Can you work these out from the model? Positions are in its coordinate system, mm. Give positions to 0.01 mm unless a question says otherwise; leave off trailing zeros. Write each loop counter-clockwise with the first axis right and the second up, starting at its lowest first coordinate (ties: lowest second). Pieces come first, ordered by that corner, then holes.
```python
from build123d import *

# Parameters (mm, degrees)
SKETCH1_W           = 155
SKETCH1_H           = 110
BOSS_EXTRUDE1_DEPTH = 80
SKETCH2_W           = 151
SKETCH2_H           = 106
CUT_EXTRUDE1_DEPTH  = 78
SKETCH3_R           = 2.5
CUT_EXTRUDE2_DEPTH  = 2
SKETCH7_R           = 1.6
CUT_EXTRUDE7_DEPTH  = 2
SKETCH4_W           = 27.5
SKETCH4_H           = 46.8
CUT_EXTRUDE8_DEPTH  = 2
SKETCH8_W           = 4
SKETCH8_H           = 53
CUT_EXTRUDE9_DEPTH  = 2
SKETCH9_W           = 14
SKETCH9_H           = 14
CUT_EXTRUDE10_DEPTH = 2
SKETCH10_W          = 25.2
SKETCH10_H          = 71.2
SKETCH10_R          = 1.25
CUT_EXTRUDE12_DEPTH = 2
SKETCH11_R          = 2.5
SKETCH11_R_2        = 4.5
CUT_EXTRUDE13_DEPTH = 2
SKETCH12_W          = 150.672892958
SKETCH12_H          = 106
SKETCH12_W_2        = 2
SKETCH12_H_2        = 110
CUT_EXTRUDE14_DEPTH = 80
SKETCH13_W          = 150.672892958
SKETCH13_H          = 2
CUT_EXTRUDE15_DEPTH = 80
SKETCH14_W          = 2
SKETCH14_H          = 106
CUT_EXTRUDE16_DEPTH = 80


with BuildPart() as part:
    # Sketch1 → Boss-Extrude1 (new body)
    with BuildSketch(Plane.XY):
        with Locations((77.5, 55)):
            Rectangle(SKETCH1_W, SKETCH1_H)
    extrude(amount=BOSS_EXTRUDE1_DEPTH)

    # Sketch2 → Cut-Extrude1 (cut)
    with BuildSketch(Plane.XY.offset(80)):
        with Locations((77.5, 55)):
            Rectangle(SKETCH2_W, SKETCH2_H)
    extrude(amount=-CUT_EXTRUDE1_DEPTH, mode=Mode.SUBTRACT)

    # Sketch3 → Cut-Extrude2 (cut)
    with BuildSketch(Plane.XY.offset(2)):
        with Locations((145, 100.5)):
            Circle(SKETCH3_R)
        with Locations((145, 9.5)):
            Circle(SKETCH3_R)
        with Locations((10, 9.5)):
            Circle(SKETCH3_R)
        with Locations((10, 100.5)):
            Circle(SKETCH3_R)
    extrude(amount=-CUT_EXTRUDE2_DEPTH, mode=Mode.SUBTRACT)

    # Sketch7 → Cut-Extrude7 (cut)
    with BuildSketch(Plane(origin=(0, 110, 0), x_dir=(1, 0, 0), z_dir=(0, 1, 0))):
        with Locations((44.48, -20.14450396)):
            Circle(SKETCH7_R)
        with Locations((95.28, -17.14)):
            Circle(SKETCH7_R)
        with Locations((95.28, -62.86)):
            Circle(SKETCH7_R)
        with Locations((44.48, -47.62)):
            Circle(SKETCH7_R)
    extrude(amount=-CUT_EXTRUDE7_DEPTH, mode=Mode.SUBTRACT)

    # Sketch4 → Cut-Extrude8 (cut)
    with BuildSketch(Plane(origin=(155, 0, 0), x_dir=(0, 0, -1), z_dir=(1, 0, 0))):
        with Locations((-40, 82.5)):
            Rectangle(SKETCH4_W, SKETCH4_H)
    extrude(amount=-CUT_EXTRUDE8_DEPTH, mode=Mode.SUBTRACT)

    # Sketch8 → Cut-Extrude9 (cut)
    with BuildSketch(Plane(origin=(155, 0, 0), x_dir=(0, 0, -1), z_dir=(1, 0, 0))):
        with Locations((-68, 28.5)):
            Rectangle(SKETCH8_W, SKETCH8_H)
        with Locations((-76, 28.5)):
            Rectangle(SKETCH8_W, SKETCH8_H)
        with Locations((-60, 28.5)):
            Rectangle(SKETCH8_W, SKETCH8_H)
        with Locations((-52, 28.5)):
            Rectangle(SKETCH8_W, SKETCH8_H)
        with Locations((-44, 28.5)):
            Rectangle(SKETCH8_W, SKETCH8_H)
        with Locations((-36, 28.5)):
            Rectangle(SKETCH8_W, SKETCH8_H)
        with Locations((-28, 28.5)):
            Rectangle(SKETCH8_W, SKETCH8_H)
        with Locations((-20, 28.5)):
            Rectangle(SKETCH8_W, SKETCH8_H)
        with Locations((-12, 28.5)):
            Rectangle(SKETCH8_W, SKETCH8_H)
        with Locations((-4, 28.5)):
            Rectangle(SKETCH8_W, SKETCH8_H)
    extrude(amount=-CUT_EXTRUDE9_DEPTH, mode=Mode.SUBTRACT)

    # Sketch9 → Cut-Extrude10 (cut)
    with BuildSketch(Plane(origin=(0, 110, 0), x_dir=(1, 0, 0), z_dir=(0, 1, 0))):
        with Locations((120, -19)):
            Rectangle(SKETCH9_W, SKETCH9_H)
    extrude(amount=-CUT_EXTRUDE10_DEPTH, mode=Mode.SUBTRACT)

    # Sketch10 → Cut-Extrude12 (cut)
    with BuildSketch(Plane.ZY):
        with Locations((58, 55)):
            Rectangle(SKETCH10_W, SKETCH10_H)
        with Locations((42.5, 92.5)):
            Circle(SKETCH10_R)
        with Locations((73.5, 92.5)):
            Circle(SKETCH10_R)
        with Locations((42.5, 17.5)):
            Circle(SKETCH10_R)
        with Locations((73.5, 17.5)):
            Circle(SKETCH10_R)
    extrude(amount=-CUT_EXTRUDE12_DEPTH, mode=Mode.SUBTRACT)

    # Sketch11 → Cut-Extrude13 (cut)
    with BuildSketch(Plane.ZY):
        with Locations((20, 55)):
            Circle(SKETCH11_R)
        with Locations((20, 40)):
            Circle(SKETCH11_R)
        with Locations((20, 25)):
            Circle(SKETCH11_R)
        with Locations((20, 82.5)):
            Circle(SKETCH11_R_2)
    extrude(amount=-CUT_EXTRUDE13_DEPTH, mode=Mode.SUBTRACT)

    # Sketch12 → Cut-Extrude14 (cut)
    with BuildSketch(Plane.XY.offset(80)):
        with Locations((77.336446479, 55)):
            Rectangle(SKETCH12_W, SKETCH12_H)
        Polygon((155, 110), (152.672892958, 110), (152.672892958, 108), (153, 108), (153, 2), (152.672892958, 2), (152.672892958, 0), (155, 0), align=None)
        with Locations((1, 55)):
            Rectangle(SKETCH12_W_2, SKETCH12_H_2)
    extrude(amount=-CUT_EXTRUDE14_DEPTH, mode=Mode.SUBTRACT)

    # Sketch13 → Cut-Extrude15 (cut)
    with BuildSketch(Plane.XY.offset(80)):
        with Locations((77.336446479, 1)):
            Rectangle(SKETCH13_W, SKETCH13_H)
    extrude(amount=-CUT_EXTRUDE15_DEPTH, mode=Mode.SUBTRACT)

    # Sketch14 → Cut-Extrude16 (cut)
    with BuildSketch(Plane(origin=(153, 0, 0), x_dir=(0, 0, -1), z_dir=(1, 0, 0))):
        with Locations((-1, 55)):
            Rectangle(SKETCH14_W, SKETCH14_H)
    extrude(amount=-CUT_EXTRUDE16_DEPTH, mode=Mode.SUBTRACT)


solid = part.part
```
1) If we mould it in two halves opening along Z, with no side actions, what happens to faces 1 (the face through (76, 108, 41)), 2 (the face through (94.93, 109.01, 64.42))? For each: +Z half, -Z half, draft (parallel to the pull), parting line (faces both ways), or undercut.
Values follow:
face 1: draft
face 2: undercut
2) Suppose I cut it at C-C on z = 17.14. Write out the boundary of the cut face in (x, y), plus the area to 3 significant figures.
Values follow:
outline: (2, 108) - (93.68, 108) - (93.68, 110) - (2, 110) - close; (96.88, 108) - (113, 108) - (113, 110) - (96.88, 110) - close; (127, 108) - (152.67, 108) - (152.67, 110) - (127, 110) - close
area: 267 mm2
3) Suppose I cut it at B-B on z = 62.86. Write out the boundary of the cut face in (x, y), plus the area to 3 significant figures.
Values follow:
outline: (2, 108) - (93.68, 108) - (93.68, 110) - (2, 110) - close; (96.88, 108) - (152.67, 108) - (152.67, 110) - (96.88, 110) - close
area: 295 mm2
4) Suppose I cut it at D-D on y = 109.65. Write out the boundary of the cut face in (x, z).
Values follow:
outline: (2, 0) - (152.67, 0) - (152.67, 80) - (2, 80) - close; hole circle Ø3.2 at (44.48, 20.14); hole circle Ø3.2 at (44.48, 47.62); hole circle Ø3.2 at (95.28, 17.14); hole circle Ø3.2 at (95.28, 62.86); hole (113, 12) - (127, 12) - (127, 26) - (113, 26) - close
5) Please list where these lines run through material, in increasing order: L1, parallel to X at y = 109.3, z = 17.14; L2, parallel to Z at x = 44.48, y = 108.7; L3, parallel to X at y = 109.25, z = 47.62.
Values follow:
L1: x = 2 to 93.68, 96.88 to 113, 127 to 152.67
L2: z = 0 to 18.54, 21.74 to 46.02, 49.22 to 80
L3: x = 2 to 42.88, 46.08 to 152.67
6) Suppose I cut it at A-A on x = 95.28. Write out the boundary of the cut face in (y, z).
Values follow:
outline: (108, 0) - (110, 0) - (110, 15.54) - (108, 15.54) - close; (108, 18.74) - (110, 18.74) - (110, 61.26) - (108, 61.26) - close; (108, 64.46) - (110, 64.46) - (110, 80) - (108, 80) - close
